CAD build for the part. Positions are in the model's coordinates, mm. A direction names the side the tool comes from. Give positions to 0.01 mm unless a question says otherwise; leave off trailing zeros. Loops run counter-clockwise (first coordinate to the right, second up) from the corner with the lowest first, then second, coordinate; pieces in that order, holes last. Notation, with made-up numbers: M 85.5,-30.5 L 130.5,-30.5 A26 ccw 130.5,-6.5 Z; hole C -19,-8 d2. An arc over 180 degrees is marked long. Answer as CSV lines item,"result".
from build123d import *

# Parameters (mm, degrees)
BOSS_EXTRUDE1_DEPTH      = 5
BOSS_EXTRUDE1_DEPTH_BACK = 7.42
SKETCH1_R                = 10
BOSS_EXTRUDE2_DEPTH      = 5


with BuildPart() as part:
    # Sketch1 → Boss-Extrude1 (new, two sides: drawn at the far end of the back side and taken through both)
    with BuildSketch(Plane.XY.offset(-BOSS_EXTRUDE1_DEPTH_BACK)):
        Circle(SKETCH1_R)
    extrude(amount=BOSS_EXTRUDE1_DEPTH + BOSS_EXTRUDE1_DEPTH_BACK)

    # Sketch2 → Boss-Extrude2 (add)
    with BuildSketch(Plane.XY.offset(5)):
        Polygon((0, 11.547005384), (-10, 5.773502692), (-10, -5.773502692), (0, -11.547005384), (10, -5.773502692), (10, 5.773502692), align=None)
    extrude(amount=BOSS_EXTRUDE2_DEPTH)


solid = part.part
1) Band-saw the part on A-A on x = 1.25. Give the cut face in (y, z).
Answer below:
outline,"M -10.83,5 L -9.92,5 L -9.92,-7.42 L 9.92,-7.42 L 9.92,5 L 10.83,5 L 10.83,10 L -10.83,10 Z"
2) Band-saw the part on D-D on z = 3. Give the cut face in (x, y), and give its area (3 significant figures).
Answer below:
outline,"C 0,0 d20"
area,"314 mm^2"
3) Flat gauge pins, fed straight in: pin 1 (2 mm diameter, centred on y = -2.5, z = 2.5, fed in from -X); pin 2 (8 mm diameter, centred on y = -7.5, z = -0.5, fed in from +X); pin 3 (4 mm diameter, centred on x = -2.5, z = 5, fed in from -Y). Where does each tip first touch, or does it go through?
Answer below:
pin 1,"stops at x = -9.89"
pin 2,"stops at x = 9.37"
pin 3,"stops at y = -11.26"
4) Which spindle directions (+Z, -Z, +X, -X, +Y, -Y) get a long thin tool onto all of the face, cutting with end or side? Do faces 1 (the face through (-9, 5, 5)), 2 (the face through (9, 5, 5)), 3 (the face through (0, -10.3, 5)). Say none if no direction does.
Answer below:
face 1,"-Z, -X, +Y"
face 2,"-Z, +X, +Y"
face 3,"-Z, -Y"
5) Band-saw the part on C-C on y = 7.75. Give the cut face in (x, z), and give its area (3 significant figures).
Answer below:
outline,"M -6.58,5 L -6.32,5 L -6.32,-7.42 L 6.32,-7.42 L 6.32,5 L 6.58,5 L 6.58,10 L -6.58,10 Z"
area,"223 mm^2"
6) Band-saw the part on B-B on z = 7. Give the cut face in (x, y), and give its area (3 significant figures).
Answer below:
outline,"M -10,-5.77 L 0,-11.55 L 10,-5.77 L 10,5.77 L 0,11.55 L -10,5.77 Z"
area,"346 mm^2"
7) Drill centre lines: line 1 (Z direction, x = 1.5, y = 10.25); line 2 (X direction, y = -7.5, z = -1.75); line 3 (X direction, y = -6.5, z = 0.75). Where is each one in solid material? Low to high. Write a range as from..to.
Answer below:
line 1,"z = 5..10"
line 2,"x = -6.61..6.61"
line 3,"x = -7.6..7.6"
